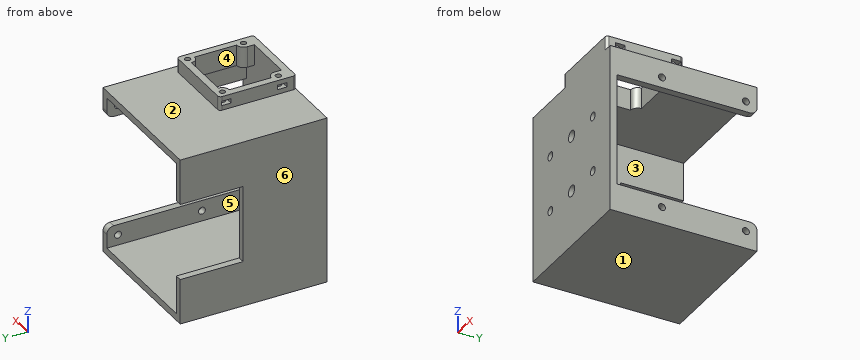
from build123d import *

# Parameters (mm, degrees)
CROQUIS1_W              = 100
CROQUIS1_H              = 120
SALIENTE_EXTRUIR1_DEPTH = 5
CORTAR_EXTRUIR5_REACH   = 80.262
CROQUIS6_R              = 3
CROQUIS6_R_2            = 4
SALIENTE_EXTRUIR2_DEPTH = 100
CROQUIS8_W              = 55
CROQUIS8_H              = 45
CORTAR_EXTRUIR6_DEPTH   = 157.923548265
CORTAR_EXTRUIR8_REACH   = 169.108
SALIENTE_EXTRUIR4_START = 10
CROQUIS13_R             = 2
SALIENTE_EXTRUIR4_DEPTH = 10
CORTAR_EXTRUIR9_DEPTH   = 1.6
CORTAR_EXTRUIR10_REACH  = 163.012
CROQUIS16_R             = 2.5
REDONDEO1_R             = 5


with BuildPart() as part:
    # Croquis1 → Saliente-Extruir1 (new body)
    with BuildSketch(Plane(origin=(0, 0, 0), x_dir=(1, 0, 0), z_dir=(0, 1, 0))):
        Rectangle(CROQUIS1_W, CROQUIS1_H)
    extrude(amount=SALIENTE_EXTRUIR1_DEPTH)

    # Croquis6 → Cortar-Extruir5 (cut, up to next)
    with BuildSketch(Plane(origin=(0, 0, 0), x_dir=(1, 0, 0), z_dir=(0, 1, 0)), mode=Mode.PRIVATE) as cortar_extruir5_sk1:
        with Locations(Location((27.5, -20, 0), (0, 0, 90))):
            Circle(CROQUIS6_R)
    cortar_extruir5_tool1 = extrude(cortar_extruir5_sk1.sketch, amount=CORTAR_EXTRUIR5_REACH, mode=Mode.PRIVATE) & part.part
    # Croquis6 → Cortar-Extruir5 (cut, up to next)
    with BuildSketch(Plane(origin=(0, 0, 0), x_dir=(1, 0, 0), z_dir=(0, 1, 0)), mode=Mode.PRIVATE) as cortar_extruir5_sk2:
        with Locations(Location((0, -20, 0), (0, 0, 90))):
            Circle(CROQUIS6_R_2)
    cortar_extruir5_tool2 = extrude(cortar_extruir5_sk2.sketch, amount=CORTAR_EXTRUIR5_REACH, mode=Mode.PRIVATE) & part.part
    # Croquis6 → Cortar-Extruir5 (cut, up to next)
    with BuildSketch(Plane(origin=(0, 0, 0), x_dir=(1, 0, 0), z_dir=(0, 1, 0)), mode=Mode.PRIVATE) as cortar_extruir5_sk3:
        with Locations(Location((-27.5, -20, 0), (0, 0, 90))):
            Circle(CROQUIS6_R)
    cortar_extruir5_tool3 = extrude(cortar_extruir5_sk3.sketch, amount=CORTAR_EXTRUIR5_REACH, mode=Mode.PRIVATE) & part.part
    # Croquis6 → Cortar-Extruir5 (cut, up to next)
    with BuildSketch(Plane(origin=(0, 0, 0), x_dir=(1, 0, 0), z_dir=(0, 1, 0)), mode=Mode.PRIVATE) as cortar_extruir5_sk4:
        with Locations(Location((-27.5, 20, 0), (0, 0, 90))):
            Circle(CROQUIS6_R)
    cortar_extruir5_tool4 = extrude(cortar_extruir5_sk4.sketch, amount=CORTAR_EXTRUIR5_REACH, mode=Mode.PRIVATE) & part.part
    # Croquis6 → Cortar-Extruir5 (cut, up to next)
    with BuildSketch(Plane(origin=(0, 0, 0), x_dir=(1, 0, 0), z_dir=(0, 1, 0)), mode=Mode.PRIVATE) as cortar_extruir5_sk5:
        with Locations(Location((0, 20, 0), (0, 0, 90))):
            Circle(CROQUIS6_R_2)
    cortar_extruir5_tool5 = extrude(cortar_extruir5_sk5.sketch, amount=CORTAR_EXTRUIR5_REACH, mode=Mode.PRIVATE) & part.part
    # Croquis6 → Cortar-Extruir5 (cut, up to next)
    with BuildSketch(Plane(origin=(0, 0, 0), x_dir=(1, 0, 0), z_dir=(0, 1, 0)), mode=Mode.PRIVATE) as cortar_extruir5_sk6:
        with Locations(Location((27.5, 20, 0), (0, 0, 90))):
            Circle(CROQUIS6_R)
    cortar_extruir5_tool6 = extrude(cortar_extruir5_sk6.sketch, amount=CORTAR_EXTRUIR5_REACH, mode=Mode.PRIVATE) & part.part
    add(cortar_extruir5_tool1.solids().sort_by_distance((27.5, 0, 20))[0], mode=Mode.SUBTRACT)
    add(cortar_extruir5_tool2.solids().sort_by_distance((0, 0, 20))[0], mode=Mode.SUBTRACT)
    add(cortar_extruir5_tool3.solids().sort_by_distance((-27.5, 0, 20))[0], mode=Mode.SUBTRACT)
    add(cortar_extruir5_tool4.solids().sort_by_distance((-27.5, 0, -20))[0], mode=Mode.SUBTRACT)
    add(cortar_extruir5_tool5.solids().sort_by_distance((0, 0, -20))[0], mode=Mode.SUBTRACT)
    add(cortar_extruir5_tool6.solids().sort_by_distance((27.5, 0, -20))[0], mode=Mode.SUBTRACT)

    # Croquis7 → Saliente-Extruir2 (add)
    with BuildSketch(Plane(origin=(0, 5, 0), x_dir=(1, 0, 0), z_dir=(0, 1, 0))):
        Polygon((45, 40), (50, 40), (50, 60), (-50, 60), (-50, -60), (50, -60), (50, -40), (45, -40), (45, -55), (-45, -55), (-45, 55), (45, 55), align=None)
    extrude(amount=SALIENTE_EXTRUIR2_DEPTH)

    # Croquis8 → Cortar-Extruir6 (cut, through all)
    with BuildSketch(Plane(origin=(50, 0, 0), x_dir=(0, 0, -1), z_dir=(1, 0, 0))):
        with Locations((0, 82.5)):
            Rectangle(CROQUIS8_W, CROQUIS8_H)
    extrude(amount=-CORTAR_EXTRUIR6_DEPTH, mode=Mode.SUBTRACT)

    # Croquis12 → Cortar-Extruir8 (cut, up to next)
    with BuildSketch(Plane.XY.offset(60), mode=Mode.PRIVATE) as cortar_extruir8_sk1:
        with BuildLine():
            Line((0, 5), (35, 5))
            Line((35, 5), (35, 10))
            ThreePointArc((35, 10), (36.464466094, 13.535533906), (40, 15))
            Line((40, 15), (40, 45))
            ThreePointArc((40, 45), (36.464466094, 46.464466094), (35, 50))
            Line((35, 50), (0, 50))
            ThreePointArc((0, 50), (-1.464466094, 46.464466094), (-5, 45))
            Line((-5, 45), (-5, 15))
            ThreePointArc((-5, 15), (-1.464466094, 13.535533906), (0, 10))
            Line((0, 10), (0, 5))
        make_face()
    cortar_extruir8_tool1 = extrude(cortar_extruir8_sk1.sketch, amount=-CORTAR_EXTRUIR8_REACH, mode=Mode.PRIVATE) & part.part
    add(cortar_extruir8_tool1.solids().sort_by_distance((17.5, 27.923763, 60))[0], mode=Mode.SUBTRACT)

    # Croquis13 → Saliente-Extruir4 (add)
    with BuildSketch(Plane.XY.offset(60).offset(SALIENTE_EXTRUIR4_START)):
        with BuildLine():
            Line((-8, 0), (43, 0))
            ThreePointArc((43, 0), (44.414213562, 0.585786438), (45, 2))
            Line((45, 2), (45, 53))
            ThreePointArc((45, 53), (44.414213562, 54.414213562), (43, 55))
            Line((43, 55), (-8, 55))
            ThreePointArc((-8, 55), (-9.414213562, 54.414213562), (-10, 53))
            Line((-10, 53), (-10, 2))
            ThreePointArc((-10, 2), (-9.414213562, 0.585786438), (-8, 0))
        make_face()
        with Locations((-5, 50)):
            Circle(CROQUIS13_R, mode=Mode.SUBTRACT)
        with Locations((40, 50)):
            Circle(CROQUIS13_R, mode=Mode.SUBTRACT)
        with Locations((40, 10)):
            Circle(CROQUIS13_R, mode=Mode.SUBTRACT)
        with Locations((-5, 10)):
            Circle(CROQUIS13_R, mode=Mode.SUBTRACT)
        with BuildLine():
            Line((0, 5), (35, 5))
            Line((35, 5), (35, 10))
            ThreePointArc((35, 10), (36.464466094, 13.535533906), (40, 15))
            Line((40, 15), (40, 45))
            ThreePointArc((40, 45), (36.464466094, 46.464466094), (35, 50))
            Line((35, 50), (0, 50))
            ThreePointArc((0, 50), (-1.464466094, 46.464466094), (-5, 45))
            Line((-5, 45), (-5, 15))
            ThreePointArc((-5, 15), (-1.464466094, 13.535533906), (0, 10))
            Line((0, 10), (0, 5))
        make_face(mode=Mode.SUBTRACT)
    extrude(amount=-SALIENTE_EXTRUIR4_DEPTH)

    # Croquis15 → Cortar-Extruir9 (cut, symmetric)
    with BuildSketch(Plane.XY.offset(65)):
        Polygon((42.020725942, 53.5), (45, 53.5), (45, 46.5), (42.020725942, 46.5), (37.979274058, 46.5), (35.958548116, 50), (37.979274058, 53.5), align=None)
        Polygon((-0.958548116, 50), (-2.979274058, 53.5), (-7.020725942, 53.5), (-10, 53.5), (-10, 46.5), (-7.020725942, 46.5), (-2.979274058, 46.5), align=None)
        Polygon((35.958548116, 10), (37.979274058, 6.5), (42.020725942, 6.5), (45, 6.5), (45, 13.5), (42.020725942, 13.5), (37.979274058, 13.5), align=None)
        Polygon((-0.958548116, 10), (-2.979274058, 13.5), (-7.020725942, 13.5), (-10, 13.5), (-10, 6.5), (-7.020725942, 6.5), (-2.979274058, 6.5), align=None)
    extrude(amount=CORTAR_EXTRUIR9_DEPTH, both=True, mode=Mode.SUBTRACT)

    # Croquis16 → Cortar-Extruir10 (cut, up to next)
    with BuildSketch(Plane(origin=(50, 0, 0), x_dir=(0, 0, -1), z_dir=(1, 0, 0)), mode=Mode.PRIVATE) as cortar_extruir10_sk1:
        with Locations((-47.5, 97)):
            Circle(CROQUIS16_R)
    cortar_extruir10_tool1 = extrude(cortar_extruir10_sk1.sketch, amount=-CORTAR_EXTRUIR10_REACH, mode=Mode.PRIVATE) & part.part
    # Croquis16 → Cortar-Extruir10 (cut, up to next)
    with BuildSketch(Plane(origin=(50, 0, 0), x_dir=(0, 0, -1), z_dir=(1, 0, 0)), mode=Mode.PRIVATE) as cortar_extruir10_sk2:
        with Locations((-47.5, 37)):
            Circle(CROQUIS16_R)
    cortar_extruir10_tool2 = extrude(cortar_extruir10_sk2.sketch, amount=-CORTAR_EXTRUIR10_REACH, mode=Mode.PRIVATE) & part.part
    # Croquis16 → Cortar-Extruir10 (cut, up to next)
    with BuildSketch(Plane(origin=(50, 0, 0), x_dir=(0, 0, -1), z_dir=(1, 0, 0)), mode=Mode.PRIVATE) as cortar_extruir10_sk3:
        with Locations((47.5, 97)):
            Circle(CROQUIS16_R)
    cortar_extruir10_tool3 = extrude(cortar_extruir10_sk3.sketch, amount=-CORTAR_EXTRUIR10_REACH, mode=Mode.PRIVATE) & part.part
    # Croquis16 → Cortar-Extruir10 (cut, up to next)
    with BuildSketch(Plane(origin=(50, 0, 0), x_dir=(0, 0, -1), z_dir=(1, 0, 0)), mode=Mode.PRIVATE) as cortar_extruir10_sk4:
        with Locations((47.5, 37)):
            Circle(CROQUIS16_R)
    cortar_extruir10_tool4 = extrude(cortar_extruir10_sk4.sketch, amount=-CORTAR_EXTRUIR10_REACH, mode=Mode.PRIVATE) & part.part
    add(cortar_extruir10_tool1.solids().sort_by_distance((50, 97, 47.5))[0], mode=Mode.SUBTRACT)
    add(cortar_extruir10_tool2.solids().sort_by_distance((50, 37, 47.5))[0], mode=Mode.SUBTRACT)
    add(cortar_extruir10_tool3.solids().sort_by_distance((50, 97, -47.5))[0], mode=Mode.SUBTRACT)
    add(cortar_extruir10_tool4.solids().sort_by_distance((50, 37, -47.5))[0], mode=Mode.SUBTRACT)

    # Redondeo1
    redondeo1_edges = [part.edges().sort_by_distance(p)[0] for p in [
        (47.5, 105, 40),
        (47.5, 105, -40),
    ]]
    fillet(redondeo1_edges, radius=REDONDEO1_R)


solid = part.part
Can you work these out from the model? Positions are in its coordinate system, mm. Face numbers are marked on the shaded views. A direction names the side the tool comes from. Coordinates: 2 decimals unless noted, no trailing zeros. Loops run counter-clockwise (first coordinate to the right, second up) from the corner with the lowest first, then second, coordinate; pieces in that order, holes last. Notation, with made-up numbers: M 5,35 L 14,35 A22 ccw 14,55 Z; hole C -37,13 d11. An arc over 180 degrees is marked long. Return JSON: item names as keys, results as strings. Group by question number.
Item 1: Imagine slicing it at C-C (y = 28). Please give me the cut outline in (x, z).
Item 2: Imagine slicing it at D-D (z = -47.5). Please give me the cut outline in (x, y), and give its area (3 significant figures).
Item 3: On a 3-axis mill with a long thin cutter (end or side, diameter ignored), from which of +Z, -Z, +X, -X, +Y, -Y can I reach the whole of each face in a straight line? I mean the marked faces 4, 5 and 6. Say none if no direction works.
Item 4: If I drill on L1, parallel to X at y = 3.4, z = -20; L2, parallel to Z at x = 40.5, y = 63; L3, parallel to Y at x = 32.5, z = 57, over which ranges is the centre line in solid material (lowest first)? Write a range as from..to.
Item 5: Thinking about a two-plate mould opening in Z: for the marked faces 1, 2 and 3, which applies, released by +Z, released by -Z, zero draft, split by the parting line, or undercut?
Item 6: I'm going to push flat-ended pins straight in: pin 1 Ø10 at (y, z) = (42, 30) entering from +X; pin 2 Ø2 at (x, z) = (-20.5, 30) entering from -Y; pin 3 Ø3.5 at (x, z) = (42, 64.5) entering from +Y; pin 4 Ø5 at (x, z) = (0, -20) entering from +Y. Where does each tip first touch, or does it pass through?
Item 7: Imagine slicing it at B-B (z = 20). Please give me the cut outline in (x, y).
Item 8: Imagine slicing it at A-A (x = 17.5). Please give me the cut outline in (y, z), and give its area (4 significant figures).
Verdict:
{
 "1": {"outline": "M -50,-60 L 50,-60 L 50,-40 L 45,-40 L 45,-55 L -45,-55 L -45,55 L -5,55 L -5,70 L -10,70 L -10,60 L -50,60 Z; M 40,55 L 45,55 L 45,40 L 50,40 L 50,60 L 45,60 L 45,70 L 40,70 Z"},
 "2": {"outline": "M -50,0 L 50,0 L 50,34.5 L 45,34.5 L 45,5 L -45,5 L -45,105 L -50,105 Z; M 45,39.5 L 50,39.5 L 50,94.5 L 45,94.5 Z; M 45,99.5 L 50,99.5 L 50,105 L 45,105 Z", "area": "1,450 mm^2"},
 "3": {"face 4": "+Z", "face 5": "+Y", "face 6": "+Z, -Z, -X, +Y, -Y"},
 "4": {"L1": "x = -50..-30.5, -24.5..-4, 4..24.5, 30.5..50", "L2": "z = -60..-55, 55..60", "L3": "y = 0..5, 50..105"},
 "5": {"face 1": "released by -Z", "face 2": "released by +Z", "face 3": "undercut"},
 "6": {"pin 1": "stops at x = -45", "pin 2": "stops at y = 0", "pin 3": "stops at y = 55", "pin 4": "passes through"},
 "7": {"outline": "M -50,0 L -30.5,0 L -30.5,5 L -45,5 L -45,60 L -50,60 Z; M -24.5,0 L -4,0 L -4,5 L -24.5,5 Z; M 4,0 L 24.5,0 L 24.5,5 L 4,5 Z; M 30.5,0 L 50,0 L 50,5 L 30.5,5 Z"},
 "8": {"outline": "M 0,-60 L 105,-60 L 105,-55 L 5,-55 L 5,70 L 0,70 Z; M 50,55 L 105,55 L 105,60 L 55,60 L 55,70 L 50,70 Z", "area": "1,475 mm^2"}
}
